Source: CAD feature listing. Evaluate the final solid. Frame: model axes, mm. Face numbers are marked on the shaded views. Round coordinates to 2 decimals unless told otherwise and drop trailing zeros. Return JSON: item names as keys, results as strings. Group by question number.
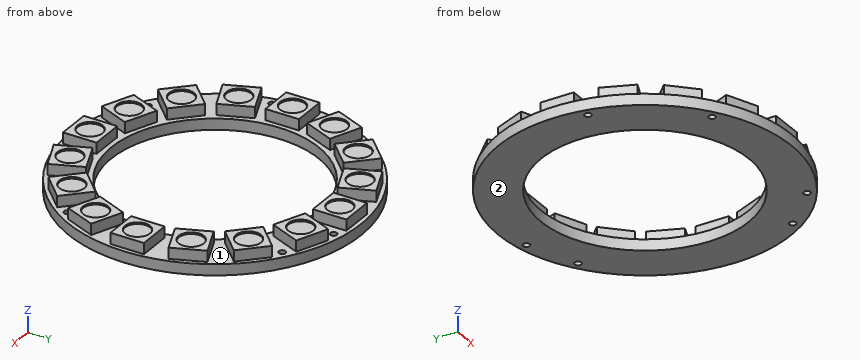
```python
from build123d import *

# Parameters (mm, degrees)
SKETCH1_R           = 22.225
SKETCH1_R_2         = 15.748
BOSS_EXTRUDE1_DEPTH = 1.6764
SKETCH2_W           = 5.08
SKETCH2_H           = 5.08
BOSS_EXTRUDE2_DEPTH = 1.6764
SKETCH3_R           = 1.905
CUT_EXTRUDE1_DEPTH  = 0.254
CIRPATTERN1_COUNT   = 16
SKETCH4_R           = 0.508
CUT_EXTRUDE2_DEPTH  = 32.475570955
CIRPATTERN2_COUNT   = 16


with BuildPart() as part:
    # Sketch1 → Boss-Extrude1 (new body)
    with BuildSketch(Plane.XY):
        Circle(SKETCH1_R)
        Circle(SKETCH1_R_2, mode=Mode.SUBTRACT)
    extrude(amount=BOSS_EXTRUDE1_DEPTH)

    # Sketch2 → Boss-Extrude2 (add)
    with BuildSketch(Plane.XY.offset(1.6764)):
        with Locations((0, 18.9865)):
            Rectangle(SKETCH2_W, SKETCH2_H)
    boss_extrude2 = extrude(amount=BOSS_EXTRUDE2_DEPTH)

    # Sketch3 → Cut-Extrude1 (cut)
    with BuildSketch(Plane.XY.offset(3.3528)):
        with Locations((0, 18.9865)):
            Circle(SKETCH3_R)
    cut_extrude1 = extrude(amount=-CUT_EXTRUDE1_DEPTH, mode=Mode.SUBTRACT)

    # CirPattern1: Boss-Extrude2, Cut-Extrude1 ×16 about axis
    cirpattern1_axis = Axis((0, 0, 0), (0, 0, 1))
    add([boss_extrude2.rotate(cirpattern1_axis, i * 360 / CIRPATTERN1_COUNT) for i in range(1, CIRPATTERN1_COUNT)])
    add([cut_extrude1.rotate(cirpattern1_axis, i * 360 / CIRPATTERN1_COUNT) for i in range(1, CIRPATTERN1_COUNT)], mode=Mode.SUBTRACT)

    # Sketch4 → Cut-Extrude2 (cut, through all)
    with BuildSketch(Plane.XY.offset(1.6764)):
        with Locations((4.088117698, 20.552355551)):
            Circle(SKETCH4_R)
    cut_extrude2 = extrude(amount=-CUT_EXTRUDE2_DEPTH, mode=Mode.SUBTRACT)

    # CirPattern2: Cut-Extrude2 ×16 about axis, 10 skipped
    cirpattern2_axis = Axis((0, 0, 0), (0, 0, 1))
    add([cut_extrude2.rotate(cirpattern2_axis, i * 360 / CIRPATTERN2_COUNT) for i in range(1, CIRPATTERN2_COUNT) if i not in (1, 2, 3, 4, 6, 8, 9, 12, 13, 14)], mode=Mode.SUBTRACT)


solid = part.part
```
(1) Cut plane C-C (z = 2.45). Count the separate pieces of the cut face and the enclosed holes in it, and give its area (3 significant figures).
(2) Pin query (flat end, axial travel): pin 1 (10 mm diameter, centred on x = -4.5, y = -12.5, fed in from +Z); pin 2 (2.5 mm diameter, centred on x = -17.54, y = -7.27, fed in from +Z); pin 3 (1.3 mm diameter, centred on y = -20, z = 2.5, fed in from -X); pin 4 (1.3 mm diameter, centred on x = 0.5, z = 2.5, fed in from +Y). Return the tip coordinate at first contact, or that it passes through.
(3) Mould query, pull axis X, two halves, no side actions, for the marked faces 1 and 2. Classes: released by +X, released by -X, zero draft, split by the parting line, or undercut.
(4) Ray query, line 1 (X direction, y = 0, z = 3.2); line 2 (X direction, y = 16.5, z = 1.85); line 3 (X direction, y = 19.5, z = 2.45). Return the intervals inside material, ascending.
Answers follow:
{
 "1": {"separate pieces": "16", "enclosed holes": "0", "area": "413 mm^2"},
 "2": {"pin 1": "z = 3.35", "pin 2": "z = 3.1", "pin 3": "x = -9.54", "pin 4": "y = 21.53"},
 "3": {"face 1": "undercut", "face 2": "zero draft"},
 "4": {"line 1": "-21.53 to -20.89, -17.08 to -16.45, 16.45 to 17.08, 20.89 to 21.53", "line 2": "-13.94 to -12.91, -9.58 to -4.09, -2.54 to 2.54, 4.09 to 9.58, 12.91 to 13.94", "line 3": "-9.17 to -5.33, -2.54 to 2.54, 5.33 to 9.17"}
}
